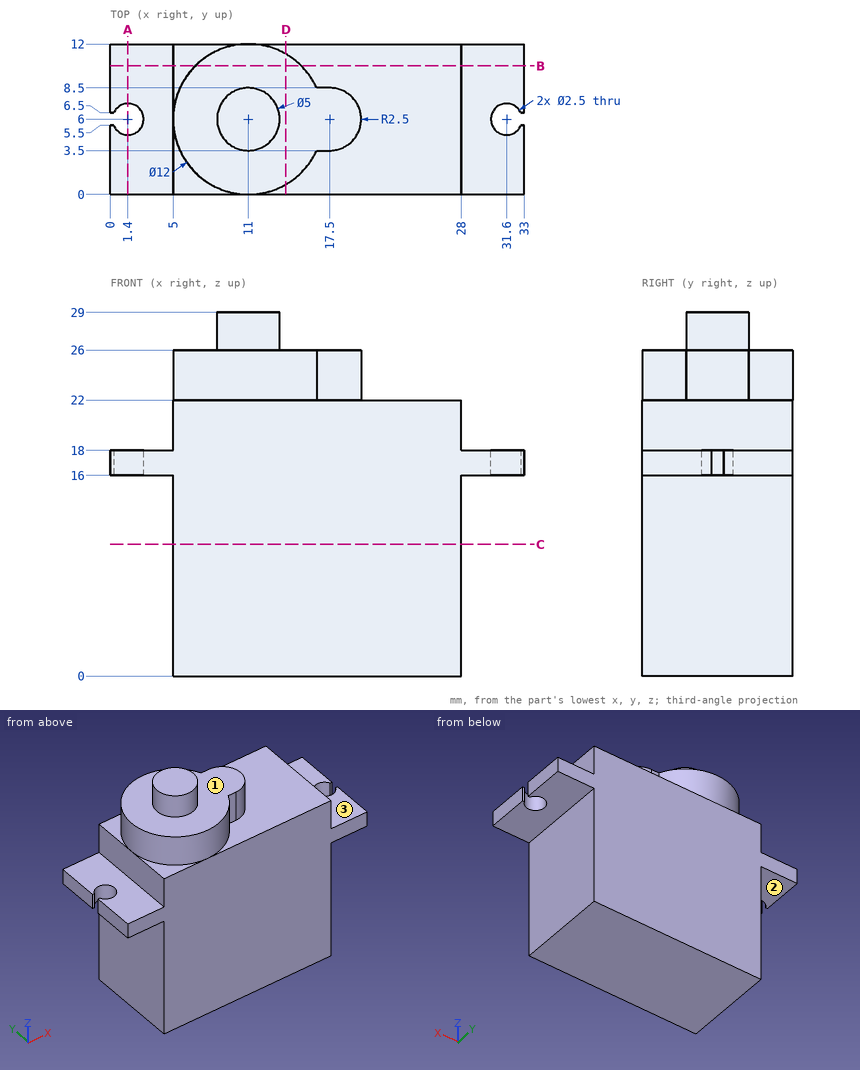
The drawing under review shows one solid part. Ordinate dimensions are in mm from its lowest x, y, z. A direction names the side the tool comes from. Coordinates: 2 decimals unless noted, no trailing zeros. Write each loop counter-clockwise with the first axis right and the second up, starting at its lowest first coordinate (ties: lowest second). Pieces come first, ordered by that corner, then holes.
1) Add section A-A (x = 1.4). Write out the cut boundary in (y, z).
2) To check wall thickness, follow L1, parallel to Y at x = 1.4, z = 16.9; L2, parallel to X at y = 6, z = 17.45; L3, parallel to Z at x = 24.5, y = 6. State the ranges of each line that lie inside material, in increasing order.
3) Machinability: for the marked faces 1, 2 and 3, which of the approach directions +Z, -Z, +X, -X, +Y, -Y give a long, thin tool a straight path to every point of the face, cutting with its end or side? Answer none if there is none.
4) Insertion check: pin 1 (3 mm diameter, centred on y = 8, z = 20.5, fed in from +X); pin 2 (2 mm diameter, centred on y = 6.5, z = 19.5, fed in from -X); pin 3 (4 mm diameter, centred on x = 1.4, y = 6, fed in from -Z). Each pin has a flat end and moves straight along its axis. Give the tip position at first contact, or say it passes through.
5) Add section D-D (x = 14). Write out the cut boundary in (y, z), plus the area to 3 significant figures.
6) Add section B-B (y = 10.25). Write out the cut boundary in (x, z), plus the area to 3 significant figures.
7) Add section C-C (z = 10.5). Write out the cut boundary in (x, y), plus the area to 3 significant figures.
Check result:
1. outline: (0, 16) - (4.75, 16) - (4.75, 18) - (0, 18) - close; (7.25, 16) - (12, 16) - (12, 18) - (7.25, 18) - close
2. L1: y = 0 to 4.75, 7.25 to 12
2. L2: x = 2.65 to 30.35
2. L3: z = 0 to 22
3. face 1: +Z
3. face 2: -Z, -X, +Y, -Y
3. face 3: +Z, +X, +Y, -Y
4. pin 1: stops at x = 28
4. pin 2: stops at x = 5
4. pin 3: stops at z = 16
5. outline: (0, 0) - (12, 0) - (12, 22) - (11.2, 22) - (11.2, 26) - (0.8, 26) - (0.8, 22) - (0, 22) - close
5. area: 306 mm2
6. outline: (0, 16) - (5, 16) - (5, 0) - (28, 0) - (28, 16) - (33, 16) - (33, 18) - (28, 18) - (28, 22) - (15.24, 22) - (15.24, 26) - (6.76, 26) - (6.76, 22) - (5, 22) - (5, 18) - (0, 18) - close
6. area: 560 mm2
7. outline: (5, 0) - (28, 0) - (28, 12) - (5, 12) - close
7. area: 276 mm2
